```python
from build123d import *

# Parameters (mm, degrees)
SKETCH1_W           = 38.1
SKETCH1_H           = 76.2
BOSS_EXTRUDE1_DEPTH = 1.27
SKETCH3_R           = 9.5
SKETCH3_R_2         = 7
BOSS_EXTRUDE2_DEPTH = 7.62
SKETCH3_5_R         = 4
CUT_EXTRUDE2_DEPTH  = 7.62
FILLET1_R           = 1.27
FILLET2_R           = 1.27


with BuildPart() as part:
    # Sketch1 → Boss-Extrude1 (new, symmetric)
    with BuildSketch(Plane(origin=(0, 0, 0), x_dir=(1, 0, 0), z_dir=(0, 1, 0))):
        with Locations((19.05, 38.1)):
            Rectangle(SKETCH1_W, SKETCH1_H)
    extrude(amount=BOSS_EXTRUDE1_DEPTH, both=True)

    # Sketch3 → Boss-Extrude2 (add)
    with BuildSketch(Plane(origin=(0, 1.27, 0), x_dir=(1, 0, 0), z_dir=(0, 1, 0))):
        with Locations(Location((19.05, 12.7, 0), (0, 0, 90))):
            Circle(SKETCH3_R)
        with Locations(Location((19.05, 12.7, 0), (0, 0, 90))):
            Circle(SKETCH3_R_2, mode=Mode.SUBTRACT)
    extrude(amount=BOSS_EXTRUDE2_DEPTH)

    # Sketch3_5 → Cut-Extrude2 (cut)
    with BuildSketch(Plane(origin=(0, 1.27, 0), x_dir=(1, 0, 0), z_dir=(0, 1, 0))):
        with Locations(Location((19.05, 12.7, 0), (0, 0, 270))):
            Circle(SKETCH3_5_R)
    extrude(amount=-CUT_EXTRUDE2_DEPTH, mode=Mode.SUBTRACT)

    # Fillet1
    fillet1_edges = [part.edges().sort_by_distance(p)[0] for p in [
        (19.05, 1.27, -3.2),
    ]]
    fillet(fillet1_edges, radius=FILLET1_R)

    # Fillet2
    fillet2_edges = [part.edges().sort_by_distance(p)[0] for p in [
        (38.1, 0, 0),
        (0, 0, 0),
    ]]
    fillet(fillet2_edges, radius=FILLET2_R)


solid = part.part
```
CAD build for the part. Positions are in the model's coordinates, mm. A direction names the side the tool comes from. Give positions to 0.01 mm unless a question says otherwise; leave off trailing zeros. Write each loop counter-clockwise with the first axis right and the second up, starting at its lowest first coordinate (ties: lowest second). Pieces come first, ordered by that corner, then holes. Notation, with made-up numbers: (86.5, -39.5) -> (137.5, -39.5) arc R18 ccw to (137.5, -29.5) -> close; hole circle Ø7 at (64, 73.5). An arc over 180 degrees is marked (long way). Write each question's results on one line, items separated by ' | '.
1. Cut at B-B, the plane z = -12.7. Write the cut outline in (x, y).
Geometry check:
outline: (0, -1.27) -> (15.05, -1.27) -> (15.05, 1.27) -> (12.05, 1.27) -> (12.05, 8.89) -> (9.55, 8.89) -> (9.55, 2.54) arc R1.27 cw to (8.28, 1.27) -> (0, 1.27) -> close; (23.05, -1.27) -> (38.1, -1.27) -> (38.1, 1.27) -> (29.82, 1.27) arc R1.27 cw to (28.55, 2.54) -> (28.55, 8.89) -> (26.05, 8.89) -> (26.05, 1.27) -> (23.05, 1.27) -> close
2. Drop flat-ended pins along their axis: P1, Ø6, axis at x = 9.5, z = -42, coming from the +Y side; P2, Ø7, axis at x = 19.05, z = -12.7, coming from the -Y side; P3, Ø6, axis at x = 8, y = 6, coming from the -Z side. Give the stop position or say it passes through.
Geometry check:
P1: y = 1.27 | P2: through | P3: z = -17.74
3. Which spindle directions (+Z, -Z, +X, -X, +Y, -Y) get a long thin tool onto all of the face, cutting with end or side? Do faces 4 (the flat face through (19, 0, -76.2)), 5 (the flat face through (22.1, 1.27, -9.7)). Say none if no direction does.
Geometry check:
face 4: -Z, +X, -X, +Y, -Y | face 5: +Y
4. Cut at A-A, the plane x = 19.05. Write the cut outline in (y, z).
Geometry check:
outline: (-1.27, -76.2) -> (1.27, -76.2) -> (1.27, -23.47) arc R1.27 cw to (2.54, -22.2) -> (8.89, -22.2) -> (8.89, -19.7) -> (1.27, -19.7) -> (1.27, -16.7) -> (-1.27, -16.7) -> close; (-1.27, -8.7) -> (1.27, -8.7) -> (1.27, -5.7) -> (8.89, -5.7) -> (8.89, -3.2) -> (2.54, -3.2) arc R1.27 cw to (1.27, -1.93) -> (1.27, 0) -> (-1.27, 0) -> close
5. Wall check: probe 1 along X at (y, z) = (3, -12.7); probe 2 along X at (y, z) = (0.75, -12.7); probe 3 along Y at (x, z) = (8.5, -4.5). Give the ranges that are in metal, low to high. Write a range as [from, to].
Geometry check:
probe 1: [9.55, 12.05], [26.05, 28.55] | probe 2: [0, 15.05], [23.05, 38.1] | probe 3: [-1.27, 1.27]
6. Cut at D-D, the plane z = -59. Write the cut outline in (x, y), then the cut area to 3 significant figures.
Geometry check:
outline: (0, -1.27) -> (38.1, -1.27) -> (38.1, 1.27) -> (0, 1.27) -> close | area: 96.8 mm²
7. Two-plate mould, pull along Z, no slides. Class faces 1 (the cylindrical face through (25.884, 5.027, -11.183)), 2 (the flat face through (19, 0, 0)), 3 (the flat face through (19, 1.27, -39)): pulls with the +Z half, pulls with the -Z half, needs draft (parallel to the pull), parting line crosses it, or undercut.
Geometry check:
face 1: undercut | face 2: pulls with the +Z half | face 3: needs draft
8. Cut at C-C, the plane y = 6.75. Write the cut outline in (x, z), then the cut area to 3 significant figures.
Geometry check:
outline: circle Ø19 at (19.05, -12.7); hole circle Ø14 at (19.05, -12.7) | area: 130 mm²
